Work out the finished part from the listing and answer in its coordinate system (mm). Face numbers are marked on the shaded views. A direction names the side the tool comes from. Give positions to 0.01 mm unless a question says otherwise; leave off trailing zeros. Order: outer loops, then holes, each group sorted by start corner. A loop starts at its lowest first (then second) coordinate and runs counter-clockwise, first axis right, second up.
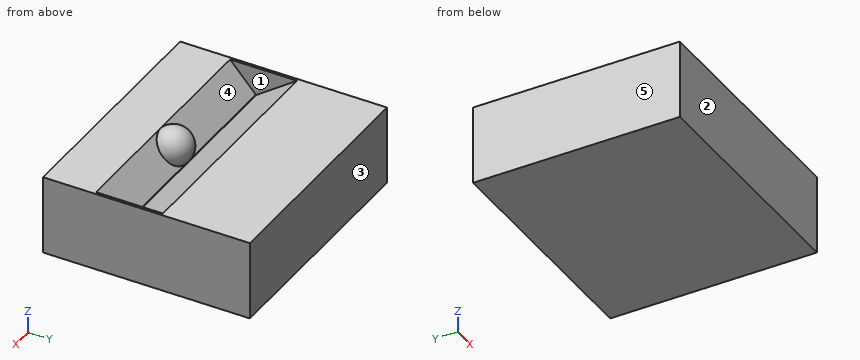
```python
from build123d import *

# Parameters (mm, degrees)
ESQUISSE1_W             = 467
ESQUISSE1_H             = 400
BOSS_EXTRU_1_DEPTH      = 153
ESQUISSE2_W             = 457
ESQUISSE2_H             = 130
ENL_V_MAT_EXTRU_1_DEPTH = 55
CHANFREIN2_SIZE2        = 78.548140371
CHANFREIN2_SIZE         = 55
CHANFREIN3_SIZE         = 50
CHANFREIN3_SIZE_2       = 55.530625741
R_VOLUTION1_ANGLE       = 182


# Some blends are built 0.0001 mm under size
with BuildPart() as part:
    # Esquisse1 → Boss.-Extru.1 (new body)
    with BuildSketch(Plane.XY):
        with Locations((-32.653034301, 10.704485488)):
            Rectangle(ESQUISSE1_W, ESQUISSE1_H)
    extrude(amount=BOSS_EXTRU_1_DEPTH)

    # Esquisse2 → Enlèv. mat.-Extru.1 (cut)
    with BuildSketch(Plane.XY.offset(153)):
        with Locations((-32.653034301, -25.295514512)):
            Rectangle(ESQUISSE2_W, ESQUISSE2_H)
    extrude(amount=-ENL_V_MAT_EXTRU_1_DEPTH, mode=Mode.SUBTRACT)

    # Chanfrein2
    chanfrein2_edges = [part.edges().sort_by_distance(p)[0] for p in [
        (-32.653034301, 39.704485488, 98),
    ]]
    chanfrein2_side = [part.faces().sort_by_distance(p)[0] for p in [
        (-32.653034301, 39.704485488, 99.1),
    ]]
    chamfer(chanfrein2_edges, length=CHANFREIN2_SIZE - 0.0001, length2=CHANFREIN2_SIZE2 - 0.0001, reference=chanfrein2_side[0])  # a hair under: the kernel refuses the full size

    # Chanfrein3
    # the kernel refuses this chamfer: 55.530625741, 50 mm, written as the material it adds along each edge
    with BuildSketch(Plane(origin=(195.846965699, -90.295514512, 98), x_dir=(0, 0.9994864482690293, -0.03204434000819546), z_dir=(-1, 0, 0))) as chanfrein3_piece_1_section:
        Polygon((CHANFREIN3_SIZE * 0.999486448269, -CHANFREIN3_SIZE * 0.0320443400082), (-CHANFREIN3_SIZE_2 * 0.0320443400085, -CHANFREIN3_SIZE_2 * 0.999486448277), (0, 0), align=None)
    chanfrein3_piece_1 = extrude(amount=457, mode=Mode.PRIVATE)
    chanfrein3_piece_1 = split(chanfrein3_piece_1, bisect_by=Plane(origin=(-32.653034301, -73.821041767, 153), z_dir=(0, 0, -1)), keep=Keep.TOP, mode=Mode.PRIVATE)
    add(chanfrein3_piece_1)

    # Esquisse3 → Révolution1 (revolve)
    with BuildSketch(Plane(origin=(0, 26.477801513, 23.840719566), x_dir=(1, 0, 0), z_dir=(0, 0.7431448254773976, 0.6691306063588547))):
        with BuildLine():
            Line((-24.478047151, -173.800955084), (-24.478047151, -99.791154956))
            ThreePointArc((-24.478047151, -99.791154956), (-61.482947215, -136.79605502), (-24.478047151, -173.800955084))
        make_face()
    revolve(axis=Axis((-24.478047151, -89.817736948, 153), (0, 0.6691306063588548, -0.7431448254773975)), revolution_arc=R_VOLUTION1_ANGLE)


solid = part.part
```
1. Which of the six approach directions +Z, -Z, +X, -X, +Y, -Y give full straight-line access (tool end or side, diameter ignored) to the marked faces 1 and 2?
Findings below:
face 1: +Z
face 2: +Z, -Z, +X, -X, -Y
2. The mould has two halves that part along Y. Classify the marked faces 3, 4 and 5: pulls with the +Y half, pulls with the -Y half, needs draft (parallel to the pull), parting line crosses it, or undercut.
Findings below:
face 3: pulls with the +Y half
face 4: undercut
face 5: needs draft
3. Straight lines are drawn through the part: probe 1 along Z at (x, y) = (98.5, 106); probe 2 along Y at (x, z) = (-61.5, 106.5); probe 3 along Y at (x, z) = (113, 104). For each, find the intervals that lie inside material, in ascending order.
Findings below:
probe 1: z = 0 to 153
probe 2: y = -189.3 to -47.95, -26.7 to 210.7
probe 3: y = -189.3 to -45.7, -30.27 to 210.7
4. Given P1, Ø0.7, axis at x = 60, y = -39.5, coming from the +Z side; P2, Ø1.5, axis at x = -184, y = 45.5, coming from the +Z side; P3, Ø4, axis at x = 32.5, y = -50.5, coming from the -Z side, each flat-ended and moving along its own axis, determine where each tip first touches the part or whether it passes through.
Findings below:
P1: stops at z = 98
P2: stops at z = 153
P3: stops at z = 0
5. The part is cut by section D-D (z = 106). Write down the section's boundary in (x, y).
Findings below:
outline: (-266.15, -189.3) - (200.85, -189.3) - (200.85, 210.7) - (-266.15, 210.7) - close; hole (-261.15, -47.5) - (-50.57, -47.5) arc R31.45 cw to (1.61, -47.5) - (195.85, -47.5) - (195.85, -27.42) - (-261.15, -27.42) - close
6. The part is cut by section A-A (z = 132.5). Write down the section's boundary in (x, y).
Findings below:
outline: (-266.15, -189.3) - (200.85, -189.3) - (200.85, 210.7) - (-266.15, 210.7) - close; hole (-261.15, -71.36) - (-60.26, -71.36) arc R36.34 cw (long way) to (11.31, -71.36) - (195.85, -71.36) - (195.85, 10.43) - (-261.15, 10.43) - close
7. The part is cut by section C-C (y = 12). Write down the section's boundary in (x, z).
Findings below:
outline: (-266.15, 0) - (200.85, 0) - (200.85, 153) - (195.85, 153) - (195.85, 133.6) - (-261.15, 133.6) - (-261.15, 153) - (-266.15, 153) - close
